Source: three-view drawing plus pictorial views. Frame: mm from the lowest corner of the part. A direction names the side the tool comes from. Give positions to 0.01 mm unless a question says otherwise; leave off trailing zeros. Order: outer loops, then holes, each group sorted by start corner. A loop starts at its lowest first (then second) coordinate and runs counter-clockwise, first axis right, second up. Notation, with made-up numbers: (-25.75, 14.25) -> (-8.75, 14.25) arc R7 cw to (-8.75, 19.25) -> close; hole circle Ø5 at (-18, -11.75). An arc over 180 degrees is marked (long way). Answer in a Markdown table with one row per item.
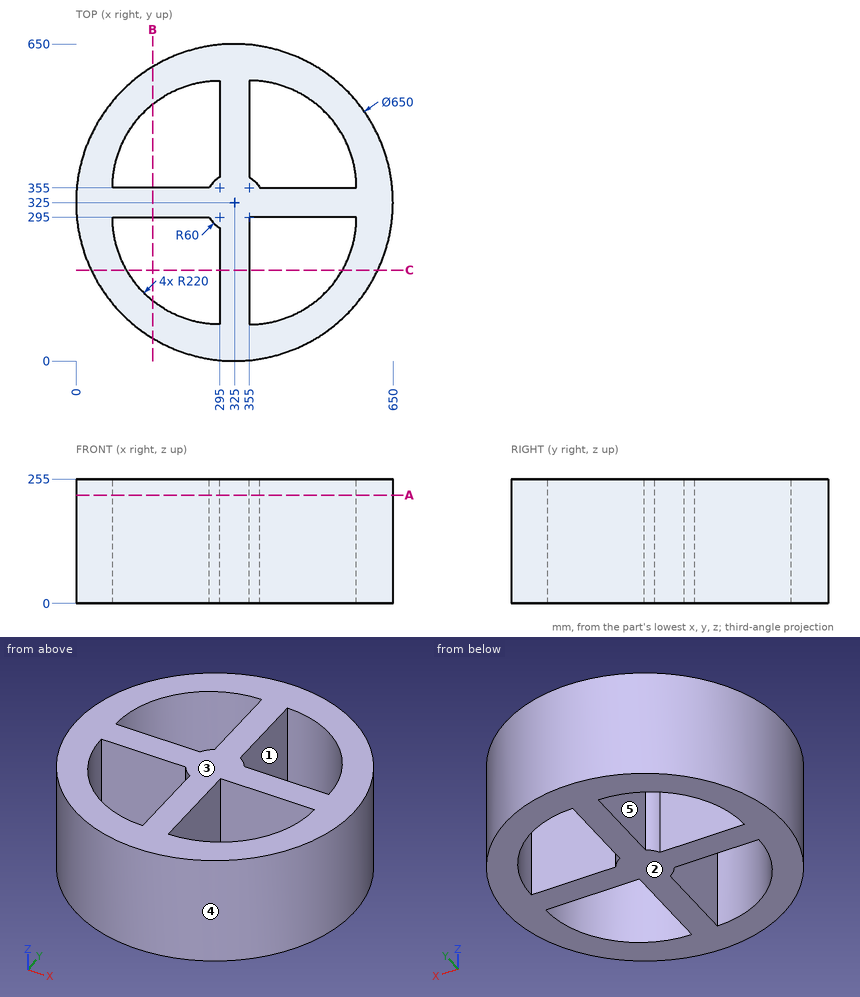
(1) Pull-direction query (Y, two-part tool) for the marked faces 3, 4 and 5; classes: +Y half, -Y half, draft (parallel to the pull), parting line (faces both ways), or undercut.
A:
| item | result |
|---|---|
| face 3 | draft |
| face 4 | parting line |
| face 5 | undercut |
(2) First-contact query: pin 1 Ø12 at (y, z) = (579, 40.5) entering from +X; pin 2 Ø4 at (y, z) = (515, 36) entering from +X; pin 3 Ø4 at (x, z) = (263, 82) entering from -Y. Flat tips, straight axial feed; report the tip coordinate or a pass-through.
A:
| item | result |
|---|---|
| pin 1 | stops at x = 535.05 |
| pin 2 | stops at x = 590.11 |
| pin 3 | stops at y = 5.59 |
(3) Ray query, probe 1 along X at (y, z) = (460, 63); probe 2 along Y at (x, z) = (188.5, 62); probe 3 along Y at (x, z) = (474, 113.5). Return the intervals inside material, ascending.
A:
| item | result |
|---|---|
| probe 1 | x = 29.37 to 101.67, 295 to 355, 548.33 to 620.63 |
| probe 2 | y = 30.05 to 102.5, 295 to 355, 547.5 to 619.95 |
| probe 3 | y = 36.17 to 109.96, 295 to 355, 540.04 to 613.83 |
(4) Section query A-A (z = 222). Return the cut outline in (x, y).
A:
| item | result |
|---|---|
| outline | circle Ø650 at (325, 325); hole (75, 295) arc R220 ccw to (295, 75) -> (295, 273.04) arc R60 cw to (273.04, 295) -> close; hole (75, 355) -> (273.04, 355) arc R60 cw to (295, 376.96) -> (295, 575) arc R220 ccw to start; hole (355, 75) arc R220 ccw to (575, 295) -> (355, 295) -> close; hole (355, 376.96) arc R60 cw to (376.96, 355) -> (575, 355) arc R220 ccw to (355, 575) -> close |
(5) Access query for the marked faces 1 and 2. Directions: +Z, -Z, +X, -X, +Y, -Y. A direction counts if a zero-diameter tool reaches every point of the face in a straight line with its end or side. Return the directions, or none.
A:
| item | result |
|---|---|
| face 1 | +Z, -Z |
| face 2 | -Z, +X, -X, +Y, -Y |
(6) Section query C-C (y = 186.5). Return the cut outline in (x, z), plus the area to 3 significant figures.
A:
| item | result |
|---|---|
| outline | (30.99, 0) -> (103.62, 0) -> (103.62, 255) -> (30.99, 255) -> close; (295, 0) -> (355, 0) -> (355, 255) -> (295, 255) -> close; (546.38, 0) -> (619.01, 0) -> (619.01, 255) -> (546.38, 255) -> close |
| area | 52,300 mm^2 |
(7) Section query B-B (x = 157). Return the cut outline in (y, z).
A:
| item | result |
|---|---|
| outline | (46.79, 0) -> (123.66, 0) -> (123.66, 255) -> (46.79, 255) -> close; (295, 0) -> (355, 0) -> (355, 255) -> (295, 255) -> close; (526.34, 0) -> (603.21, 0) -> (603.21, 255) -> (526.34, 255) -> close |
